Source: three-view drawing plus pictorial views. Frame: mm from the lowest corner of the part. Give positions to 0.01 mm unless a question says otherwise; leave off trailing zeros. Order: outer loops, then holes, each group sorted by start corner. A loop starts at its lowest first (then second) coordinate and runs counter-clockwise, first axis right, second up.
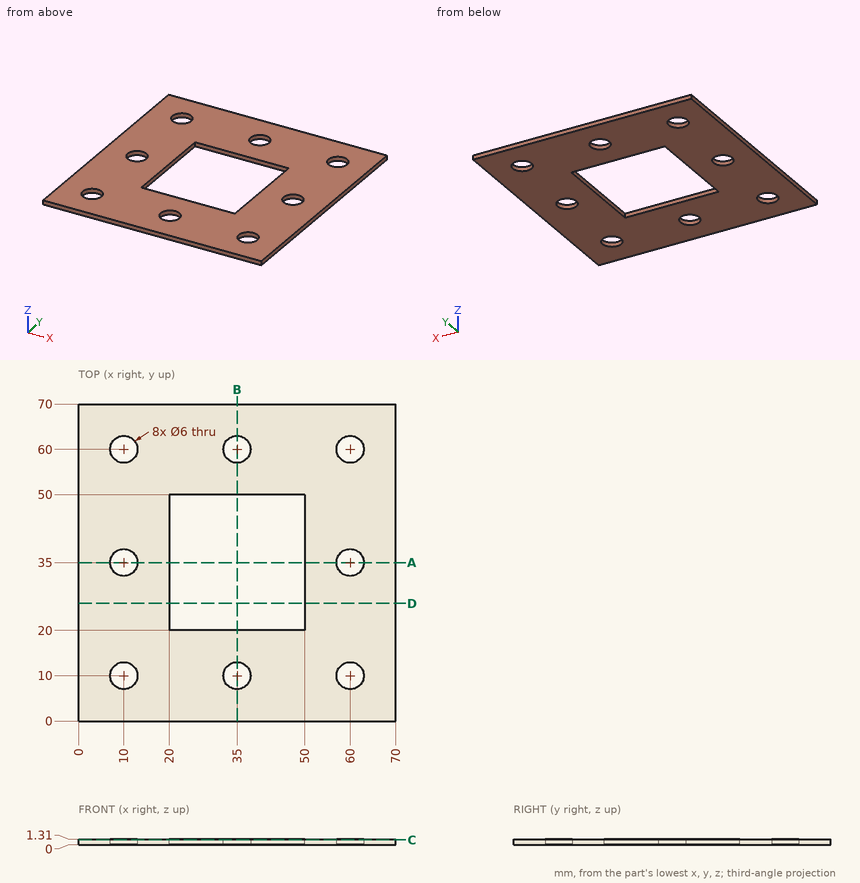
1) Section query D-D on y = 26. Output: boundary loops of the cut face in (x, z), and give its area (3 significant figures).
Checks:
outline: (0, 0) - (20, 0) - (20, 1.31) - (0, 1.31) - close; (50, 0) - (70, 0) - (70, 1.31) - (50, 1.31) - close
area: 52.4 mm2
2) Ray query, L1, parallel to Y at x = 10, z = 0.45; L2, parallel to X at y = 26, z = 0.6. Return the intervals inside material, ascending.
Checks:
L1: y = 0 to 7, 13 to 32, 38 to 57, 63 to 70
L2: x = 0 to 20, 50 to 70
3) First-contact query: pin 1 Ø4 at (x, y) = (59.5, 13.5) entering from -Z. Flat tip, straight axial feed; report the tip coordinate or a pass-through.
Checks:
pin 1: stops at z = 0
4) Section query C-C on z = 1.1. State how many separate pieces and enclosed holes the cut face has, and give its area (3 significant figures).
Checks:
separate pieces: 1
enclosed holes: 9
area: 3,770 mm2
5) Section query A-A on y = 35. Output: boundary loops of the cut face in (x, z), and give its area (3 significant figures).
Checks:
outline: (0, 0) - (7, 0) - (7, 1.31) - (0, 1.31) - close; (13, 0) - (20, 0) - (20, 1.31) - (13, 1.31) - close; (50, 0) - (57, 0) - (57, 1.31) - (50, 1.31) - close; (63, 0) - (70, 0) - (70, 1.31) - (63, 1.31) - close
area: 36.7 mm2
